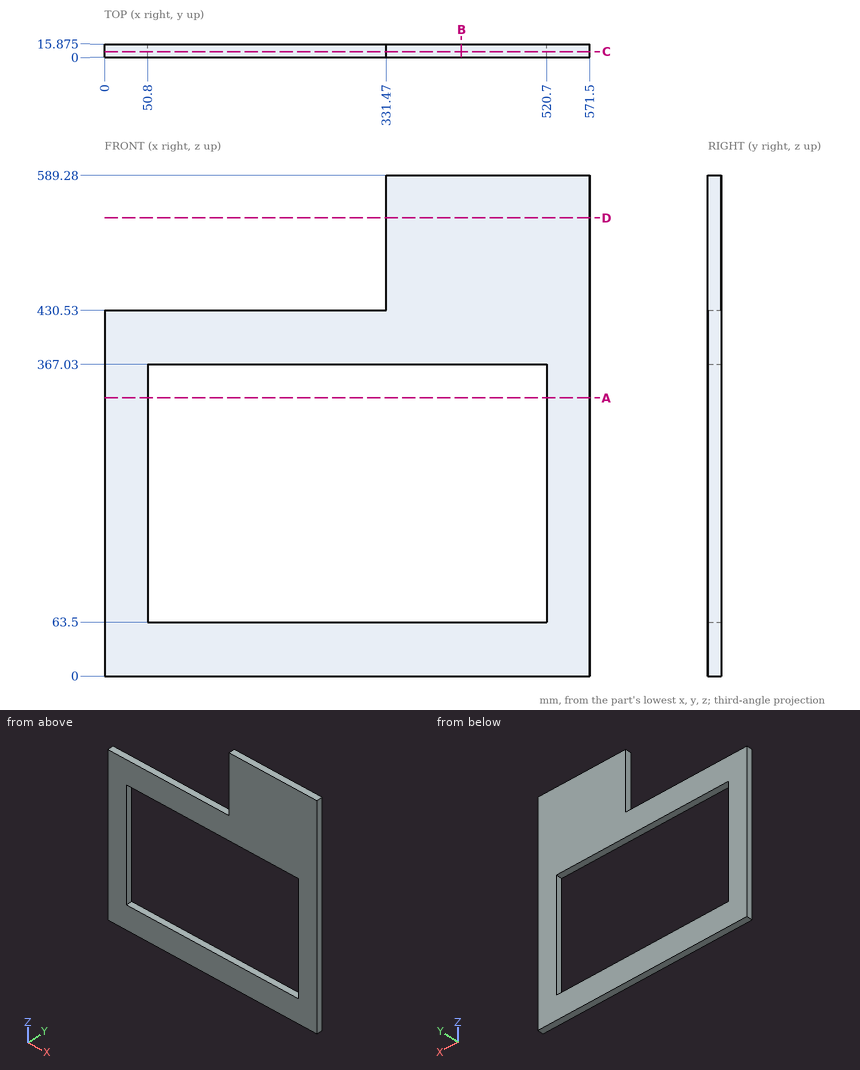
Could you check a few things on this drawing? It's one solid part, dimensions in mm from its lowest x, y, z. Give positions to 0.01 mm unless a question says otherwise; leave off trailing zeros. Write each loop counter-clockwise with the first axis right and the second up, starting at its lowest first coordinate (ties: lowest second). Pieces come first, ordered by that corner, then holes. Notation, with made-up numbers: (-37, 66.5) -> (9, 66.5) arc R32 cw to (9, 95.5) -> close; hole circle Ø10 at (-37, 55). An arc over 180 degrees is marked (long way). Write each question's results on one line, items separated by ' | '.
1. I want a section at A-A, the plane z = 327.5. Write out the boundary of the cut face in (x, y) (3 decimals).
Check sheet entries:
outline: (0, 0) -> (50.8, 0) -> (50.8, 15.875) -> (0, 15.875) -> close; (520.7, 0) -> (571.5, 0) -> (571.5, 15.875) -> (520.7, 15.875) -> close
2. I need wall thicknesses on L1, parallel to Z at x = 173.5, y = 8.5; L2, parallel to Z at x = 365, y = 15.25; L3, parallel to X at y = 13.5, z = 286.5. Which ranges of each line are inside material? Lowest first, please.
Check sheet entries:
L1: z = 0 to 63.5, 367.03 to 430.53 | L2: z = 0 to 63.5, 367.03 to 589.28 | L3: x = 0 to 50.8, 520.7 to 571.5
3. I want a section at B-B, the plane x = 420. Write out the boundary of the cut face in (y, z) (3 decimals), then the cut area to 3 significant figures.
Check sheet entries:
outline: (0, 0) -> (15.875, 0) -> (15.875, 63.5) -> (0, 63.5) -> close; (0, 367.03) -> (15.875, 367.03) -> (15.875, 589.28) -> (0, 589.28) -> close | area: 4,540 mm²
4. I want a section at D-D, the plane z = 539.5. Write out the boundary of the cut face in (x, y) (3 decimals).
Check sheet entries:
outline: (331.47, 0) -> (571.5, 0) -> (571.5, 15.875) -> (331.47, 15.875) -> close
5. Will these pins go through, and if not, where does the flat tip stop? pin 1 Ø5 at (x, y) = (113, 13) entering from +Z; pin 2 Ø1.5 at (x, z) = (455, 366.5) entering from -Y; pin 3 Ø8 at (y, z) = (10, 498.5) entering from -X.
Check sheet entries:
pin 1: stops at z = 430.53 | pin 2: stops at y = 0 | pin 3: stops at x = 331.47
6. I want a section at C-C, the plane y = 7. Write out the boundary of the cut face in (x, z), then the cut area to 3 significant figures.
Check sheet entries:
outline: (0, 0) -> (571.5, 0) -> (571.5, 589.28) -> (331.47, 589.28) -> (331.47, 430.53) -> (0, 430.53) -> close; hole (50.8, 63.5) -> (520.7, 63.5) -> (520.7, 367.03) -> (50.8, 367.03) -> close | area: 142,000 mm²
